Input: part model. Units: mm. Frame: model coordinates. Give positions to 0.01 mm unless a question says otherwise; leave off trailing zeros. Write each loop counter-clockwise with the first axis right and the second up, starting at its lowest first coordinate (ties: lowest second). Pieces come first, ordered by that corner, then holes. Notation, with made-up numbers: (-36.5, 22) - (14.5, 22) arc R21 cw to (14.5, 39) - close; hole circle Ø7 at (78.25, 43.5). An arc over 180 degrees is marked (long way). Use a Markdown table: item, result. Add a question column.
1. Pin query (flat end, axial travel): pin 1 (12 mm diameter, centred on x = 18.5, y = 4.5, fed in from -Z); pin 2 (2.5 mm diameter, centred on x = -11, y = 0, fed in from +Z); pin 3 (0.9 mm diameter, centred on x = -5, z = 2, fed in from +Y); pin 4 (1 mm diameter, centred on x = 16, z = 2, fed in from +Y). Return the tip coordinate at first contact, or that it passes through.
2. Section query D-D, the plane y = 2.75. Return loops of the section in (x, z).
3. Section query C-C, the plane x = 2.5. Return loops of the section in (y, z).
4. Material intervals for probe 1 along Y at (x, z) = (-11, 0.8); probe 2 along X at (y, z) = (-0.75, 1.7); probe 3 along Y at (x, z) = (-7.5, 0.7), sorted ascending.
5. Section query B-B, the plane y = 0. Return loops of the section in (x, z).
6. Section query A-A, the plane z = 2.55. Return loops of the section in (x, y), plus the area to 3 significant figures.
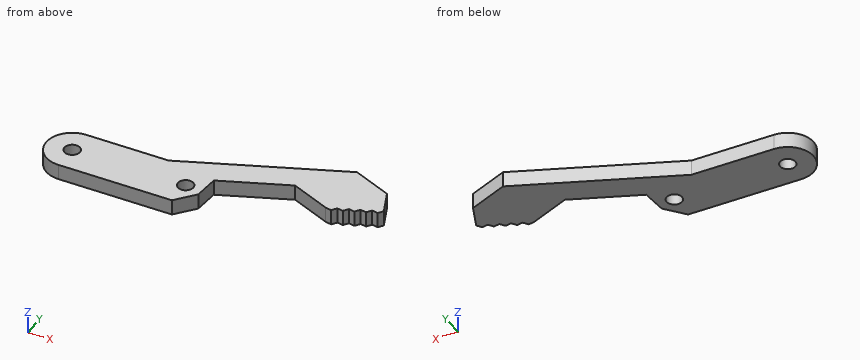
```python
from build123d import *

# Parameters (mm, degrees)
SKETCH2_R               = 1.5
BOSS_EXTRUDE1_DEPTH     = 3
BOSS_EXTRUDE2_DEPTH     = 3
CUT_EXTRUDE1_DEPTH      = 3
CUT_EXTRUDE2_DEPTH      = 1
CUT_EXTRUDE2_DEPTH_BACK = 4


with BuildPart() as part:
    # Sketch2 → Boss-Extrude1 (new body)
    with BuildSketch(Plane.XY):
        with BuildLine():
            Line((11, 5), (-11, 5))
            ThreePointArc((-11, 5), (-16, 0), (-11, -5))
            Line((-11, -5), (11, -5))
            ThreePointArc((11, -5), (16, 0), (11, 5))
        make_face()
        with Locations((-11, 0)):
            Circle(SKETCH2_R, mode=Mode.SUBTRACT)
        with Locations((11, 0)):
            Circle(SKETCH2_R, mode=Mode.SUBTRACT)
    extrude(amount=BOSS_EXTRUDE1_DEPTH)

    # Sketch3 → Boss-Extrude2 (add)
    with BuildSketch(Plane.XY.offset(3)):
        with BuildLine():
            Line((44.729340863, 8.668642725), (35.461430272, 4.9128694))
            Line((35.461430272, 4.9128694), (35.224816552, 5.496747767))
            Line((35.224816552, 5.496747767), (27.564491501, 8.738899793))
            Line((27.564491501, 8.738899793), (14.589416673, 3.480817138))
            ThreePointArc((14.589416673, 3.480817138), (12.94883482, 4.604567607), (11, 5))
            Line((11, 5), (5.025381266, 5))
            Line((5.025381266, 5), (40.405753968, 19.337714926))
            Line((40.405753968, 19.337714926), (44.729340863, 8.668642725))
        make_face()
    extrude(amount=-BOSS_EXTRUDE2_DEPTH)

    # Sketch5 → Cut-Extrude1 (cut)
    with BuildSketch(Plane.XY.offset(3)):
        Polygon((40.405753968, 19.337714926), (42.567547416, 14.003178826), (35.071217868, 17.175921479), align=None)
    extrude(amount=-CUT_EXTRUDE1_DEPTH, mode=Mode.SUBTRACT)

    # Sketch6 → Cut-Extrude2 (cut, two sides)
    with BuildSketch(Plane.XY.offset(3)) as cut_extrude2_sk:
        Polygon((40.785562907, 7.750211762), (40.095385567, 6.790756063), (41.948967686, 7.541910728), align=None)
        Polygon((38.931980789, 6.999057097), (38.241803449, 6.039601398), (40.095385567, 6.790756063), align=None)
        Polygon((37.078398671, 6.247902432), (36.388221331, 5.288446733), (38.241803449, 6.039601398), align=None)
        Polygon((36.388221331, 5.288446733), (35.224816552, 5.496747767), (35.461430272, 4.9128694), align=None)
        Polygon((42.639145025, 8.501366427), (41.948967686, 7.541910728), (43.802549804, 8.293065393), align=None)
        Polygon((44.492727144, 9.252521092), (43.802549804, 8.293065393), (44.729340863, 8.668642725), align=None)
        with BuildLine():
            ThreePointArc((11, -5), (15.604567607, -1.94883482), (14.589416673, 3.480817138))
            Line((14.589416673, 3.480817138), (14.167937437, -1.340796208))
            Line((14.167937437, -1.340796208), (11, -5))
        make_face()
    extrude(amount=CUT_EXTRUDE2_DEPTH, mode=Mode.SUBTRACT)
    extrude(cut_extrude2_sk.sketch, amount=-CUT_EXTRUDE2_DEPTH_BACK, mode=Mode.SUBTRACT)


solid = part.part
```
Result sheet:
| question | item | result |
|---|---|---|
| 1 | pin 1 | stops at z = 0 |
| 1 | pin 2 | passes through |
| 1 | pin 3 | stops at y = 5 |
| 1 | pin 4 | stops at y = 9.65 |
| 2 | outline | (-15.18, 0) - (14.53, 0) - (14.53, 3) - (-15.18, 3) - close |
| 3 | outline | (-5, 0) - (5, 0) - (5, 3) - (-5, 3) - close |
| 4 | probe 1 | y = -5 to -1.5, 1.5 to 5 |
| 4 | probe 2 | x = -15.94 to -12.3, -9.7 to 9.7, 12.3 to 14.22 |
| 4 | probe 3 | y = -5 to 5 |
| 5 | outline | (-16, 0) - (-12.5, 0) - (-12.5, 3) - (-16, 3) - close; (-9.5, 0) - (9.5, 0) - (9.5, 3) - (-9.5, 3) - close; (12.5, 0) - (14.29, 0) - (14.29, 3) - (12.5, 3) - close |
| 6 | outline | (-11, -5) - (11, -5) - (14.17, -1.34) - (14.59, 3.48) - (27.56, 8.74) - (35.22, 5.5) - (36.39, 5.29) - (37.08, 6.25) - (38.24, 6.04) - (38.93, 7) - (40.1, 6.79) - (40.79, 7.75) - (41.95, 7.54) - (42.64, 8.5) - (43.8, 8.29) - (44.49, 9.25) - (42.57, 14) - (35.07, 17.18) - (5.03, 5) - (-11, 5) arc R5 ccw to start; hole circle Ø3 at (-11, 0); hole circle Ø3 at (11, 0) |
| 6 | area | 498 mm² |
